The listing builds one solid part. Answer for the finished solid, in the listing's coordinates (mm). A direction names the side the tool comes from. Give positions to 0.01 mm unless a question says otherwise; leave off trailing zeros. Write each loop counter-clockwise with the first axis right and the second up, starting at its lowest first coordinate (ties: lowest second). Pieces come first, ordered by that corner, then holes. Notation, with made-up numbers: M 35.5,44 L 42.5,44 A26 ccw 42.5,68 Z; hole C -4.75,59 d10. An arc over 180 degrees is marked long. Answer as a JSON object with one key per item and string values.
```python
from build123d import *

# Parameters (mm, degrees)
SKETCH1_R           = 1
BOSS_EXTRUDE2_DEPTH = 5
FILLET1_R           = 0.75


with BuildPart() as part:
    # Sketch1 → Boss-Extrude2 (new body)
    with BuildSketch(Plane(origin=(0, 0, 0), x_dir=(1, 0, 0), z_dir=(0, 1, 0))):
        with BuildLine():
            Line((-1.136805092, 2.066410525), (-0.613869143, 0.60302827))
            ThreePointArc((-0.613869143, 0.60302827), (0.35214746, -0.005581798), (1.492263995, -0.066643898))
            Line((1.492263995, -0.066643898), (15.923799424, 3.58412039))
            ThreePointArc((15.923799424, 3.58412039), (19.413112634, 6.553816474), (23.917744363, 5.715547725))
            Line((23.917744363, 5.715547725), (28.235048802, 6.73364228))
            Line((28.235048802, 6.73364228), (40.313961493, 0.074349637))
            Line((40.313961493, 0.074349637), (48.41423182, -1.403905787))
            ThreePointArc((48.41423182, -1.403905787), (50.149589372, -1.191061521), (51.226168842, 0.186525195))
            Line((51.226168842, 0.186525195), (51.441108403, 1.760534064))
            ThreePointArc((51.441108403, 1.760534064), (51.382015555, 2.083995414), (51.185428041, 2.34757189))
            Line((51.185428041, 2.34757189), (39.388940164, 4.548224923))
            Line((39.388940164, 4.548224923), (37.817705686, 11.041835021))
            Line((37.817705686, 11.041835021), (37.66842193, 11.65879609))
            Line((37.66842193, 11.65879609), (37.488298502, 12.198995049))
            Line((37.488298502, 12.198995049), (37.342570627, 12.198995049))
            Line((37.342570627, 12.198995049), (24.882570627, 12.445855441))
            Line((24.882570627, 12.445855441), (22.035262293, 16.980664764))
            Line((22.035262293, 16.980664764), (10.708550227, 14.991797304))
            Line((10.708550227, 14.991797304), (10.323891999, 7.31840254))
            Line((10.323891999, 7.31840254), (-0.740858173, 3.364442041))
            ThreePointArc((-0.740858173, 3.364442041), (-1.207662762, 2.797429575), (-1.136805092, 2.066410525))
        make_face()
        with Locations((34.353341853, 5.361683953)):
            Circle(SKETCH1_R, mode=Mode.SUBTRACT)
        with Locations((45.677794697, 1.332114162)):
            Circle(SKETCH1_R, mode=Mode.SUBTRACT)
        with Locations((14.363757556, 6.840434301)):
            Circle(SKETCH1_R, mode=Mode.SUBTRACT)
        with Locations((32.086393371, 10.190351233)):
            Circle(SKETCH1_R, mode=Mode.SUBTRACT)
        with Locations((4.633423153, 2.960008936)):
            Circle(SKETCH1_R, mode=Mode.SUBTRACT)
        with Locations((16.892865834, 14.018563944)):
            Circle(SKETCH1_R, mode=Mode.SUBTRACT)
    extrude(amount=BOSS_EXTRUDE2_DEPTH)

    # Fillet1
    fillet1_edges = [part.edges().sort_by_distance(p)[0] for p in [
        (37.488298502, 2.5, -12.198995049),
        (22.035262293, 2.5, -16.980664764),
        (10.708550227, 2.5, -14.991797304),
    ]]
    fillet(fillet1_edges, radius=FILLET1_R)


solid = part.part
```
1. A cutting plane is placed at C-C, the plane x = 34. Give the vertices of the cut face in (y, z).
Verdict:
{"outline": "M 0,-12.27 L 5,-12.27 L 5,-6.3 L 0,-6.3 Z; M 0,-4.43 L 5,-4.43 L 5,-3.56 L 0,-3.56 Z"}
2. Consider line 1 along Z through (x, y) = (17, 0.4); line 2 along X through (y, z) = (1.05, -14.5); line 3 along X through (y, z) = (4.25, -10.5). Determine where each line is inside the solid, lowest interval first.
Verdict:
{"line 1": "z = -16.1 to -15.01, -13.02 to -5.15", "line 2": "x = 10.69 to 16.02, 17.77 to 23.59", "line 3": "x = 10.48 to 31.14, 33.04 to 37.95"}
3. A cutting plane is placed at B-B, the plane z = -8.5. Give the vertices of the cut face in (x, y).
Verdict:
{"outline": "M 10.38,0 L 38.43,0 L 38.43,5 L 10.38,5 Z"}
4. A cutting plane is placed at D-D, the plane y = 1.3. Count the separate pieces of the cut face and the enclosed holes in it, plus the area to 3 significant figures.
Verdict:
{"separate pieces": "1", "enclosed holes": "6", "area": "347 mm2"}
5. For faces 5 (the flat face through (34.19, 2.46, -3.45)), 6 (the flat face through (23.61, 2.46, -14.47)), determine the directions among +Z, -Z, +X, -X, +Y, -Y from which every point of the face is accessible in a straight line to the end or side of a thin tool.
Verdict:
{"face 5": "+Z, +Y, -Y", "face 6": "-Z, +X, +Y, -Y"}
6. A cutting plane is placed at A-A, the plane x = 46. Give the vertices of the cut face in (y, z).
Verdict:
{"outline": "M 0,-3.31 L 5,-3.31 L 5,-2.28 L 0,-2.28 Z; M 0,-0.39 L 5,-0.39 L 5,0.96 L 0,0.96 Z"}
7. The mould has two halves that part along Z. Classify faces 1 (the flat face through (4.87, 2.46, -5.37)), 2 (the cylindrical face through (35.307, 2.465, -5.662)), 3 (the flat face through (25, 0, -8)), 4 (the cylindrical face through (5.09, 2.46, -2.07)): released by +Z, released by -Z, zero draft, split by the parting line, or undercut.
Verdict:
{"face 1": "released by -Z", "face 2": "undercut", "face 3": "zero draft", "face 4": "undercut"}
